For this review, take the finished solid that the model builds, in its own axes (mm). Face numbers are marked on the shaded views. A direction names the side the tool comes from. Coordinates: 2 decimals unless noted, no trailing zeros. Write each loop counter-clockwise with the first axis right and the second up, starting at its lowest first coordinate (ties: lowest second). Pieces come first, ordered by that corner, then holes.
1) We need section B-B on x = 40. Write out the cut boundary in (y, z).
2) Insertion check: P1, Ø5, axis at x = 164.5, y = 26.5, coming from the -Z side; P2, Ø5, axis at x = 167, z = 41.5, coming from the +Y side; P3, Ø3, axis at x = 5.5, y = 27, coming from the +Z side. Each pin has a flat end and moves straight along its axis. Give the tip position at first contact, or say it passes through.
3) For the marked faces 1 and 2, list the 3-axis set-ups (+Z, -Z, +X, -X, +Y, -Y) from which the entire face can be reached by the end or side of a thin tool; tool diameter is ignored.
4) We need section D-D on x = 109. Write out the cut boundary in (y, z), then the cut area to 3 significant figures.
5) Mouldability with a two-part tool opening along X and no side actions: class the marked faces 3, 4 and 5 as pulls with the +X half, pulls with the -X half, needs draft (parallel to the pull), parting line crosses it, or undercut.
6) To check wall thickness, follow line 1 along X through (y, z) = (87.5, 41); line 2 along Y through (x, z) = (120, 45). State the ranges of each line that lie inside material, in increasing order.
7) We need section A-A on y = 109. Write out the cut boundary in (x, z), then the cut area to 3 significant figures.
8) We need section C-C on z = 53. Write out the cut boundary in (x, y).
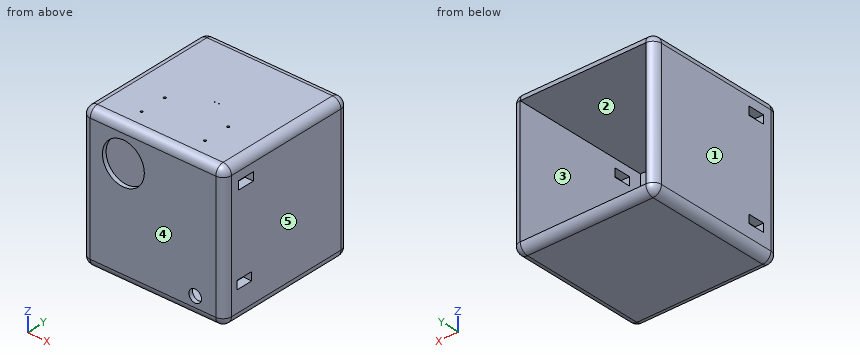
from build123d import *

# Parameters (mm, degrees)
SKETCH1_W           = 170
SKETCH1_H           = 170
BOSS_EXTRUDE2_DEPTH = 170
FILLET5_R           = 10
SKETCH6_W           = 150
SKETCH6_H           = 150
CUT_EXTRUDE2_DEPTH  = 165
SKETCH7_R           = 25
CUT_EXTRUDE3_DEPTH  = 5
SKETCH8_R           = 0.5
CUT_EXTRUDE4_DEPTH  = 5
SKETCH9_R           = 7.5
CUT_EXTRUDE5_DEPTH  = 5
SKETCH10_R          = 1.4
CUT_EXTRUDE8_DEPTH  = 5
SKETCH19_W          = 10
SKETCH19_H          = 20
CUT_EXTRUDE12_DEPTH = 15
SKETCH14_W          = 10
SKETCH14_H          = 20
CUT_EXTRUDE15_DEPTH = 15
SKETCH14_5_W        = 10
SKETCH14_5_H        = 20
CUT_EXTRUDE16_DEPTH = 15


with BuildPart() as part:
    # Sketch1 → Boss-Extrude2 (new body)
    with BuildSketch(Plane.XY):
        with Locations((85, 85)):
            Rectangle(SKETCH1_W, SKETCH1_H)
    extrude(amount=BOSS_EXTRUDE2_DEPTH)

    # Fillet5
    fillet5_edges = [part.edges().sort_by_distance(p)[0] for p in [
        (170, 85, 170),
        (85, 170, 170),
        (0, 85, 170),
        (85, 170, 0),
        (170, 85, 0),
        (85, 0, 0),
        (0, 85, 0),
        (0, 170, 85),
        (170, 170, 85),
        (170, 0, 85),
        (0, 0, 85),
        (85, 0, 170),
    ]]
    fillet(fillet5_edges, radius=FILLET5_R)

    # Sketch6 → Cut-Extrude2 (cut)
    with BuildSketch(Plane(origin=(0, 170, 0), x_dir=(1, 0, 0), z_dir=(0, 1, 0))):
        with Locations((85, -85)):
            Rectangle(SKETCH6_W, SKETCH6_H)
    extrude(amount=-CUT_EXTRUDE2_DEPTH, mode=Mode.SUBTRACT)

    # Sketch7 → Cut-Extrude3 (cut)
    with BuildSketch(Plane(origin=(0, 0, 0), x_dir=(-1, 0, 0), z_dir=(0, -1, 0))):
        with Locations(Location((-49.635709215, -128.113207768, 0), (0, 0, 90))):
            Circle(SKETCH7_R)
    extrude(amount=-CUT_EXTRUDE3_DEPTH, mode=Mode.SUBTRACT)

    # Sketch8 → Cut-Extrude4 (cut)
    with BuildSketch(Plane.XY.offset(170)):
        with Locations((87.027102924, 82.292149715)):
            Circle(SKETCH8_R)
        with Locations((92.027102924, 82.259165374)):
            Circle(SKETCH8_R)
    extrude(amount=-CUT_EXTRUDE4_DEPTH, mode=Mode.SUBTRACT)

    # Sketch9 → Cut-Extrude5 (cut)
    with BuildSketch(Plane(origin=(0, 0, 0), x_dir=(-1, 0, 0), z_dir=(0, -1, 0))):
        with Locations(Location((-135.371528781, -22.567188871, 0), (0, 0, 90))):
            Circle(SKETCH9_R)
    extrude(amount=-CUT_EXTRUDE5_DEPTH, mode=Mode.SUBTRACT)

    # Sketch10 → Cut-Extrude8 (cut)
    with BuildSketch(Plane.XY.offset(170)):
        with Locations((48.382145487, 58.196404185)):
            Circle(SKETCH10_R)
        with Locations((123.782145487, 58.455011456)):
            Circle(SKETCH10_R)
        with Locations((48.166639428, 26.796404185)):
            Circle(SKETCH10_R)
        with Locations((123.566639428, 27.055011456)):
            Circle(SKETCH10_R)
    extrude(amount=-CUT_EXTRUDE8_DEPTH, mode=Mode.SUBTRACT)

    # Sketch19 → Cut-Extrude12 (cut)
    with BuildSketch(Plane(origin=(170, 0, 0), x_dir=(0, 0, -1), z_dir=(1, 0, 0))):
        with Locations((-40, 27.793299749)):
            Rectangle(SKETCH19_W, SKETCH19_H)
        with Locations((-145, 30)):
            Rectangle(SKETCH19_W, SKETCH19_H)
    extrude(amount=-CUT_EXTRUDE12_DEPTH, mode=Mode.SUBTRACT)

    # Sketch14 → Cut-Extrude15 (cut)
    with BuildSketch(Plane.ZY):
        with Locations((30, 30)):
            Rectangle(SKETCH14_W, SKETCH14_H)
    extrude(amount=-CUT_EXTRUDE15_DEPTH, mode=Mode.SUBTRACT)

    # Sketch14_5 → Cut-Extrude16 (cut)
    with BuildSketch(Plane.ZY):
        with Locations((30, 30)):
            Rectangle(SKETCH14_5_W, SKETCH14_5_H)
        with Locations((145, 30)):
            Rectangle(SKETCH14_5_W, SKETCH14_5_H)
    extrude(amount=-CUT_EXTRUDE16_DEPTH, mode=Mode.SUBTRACT)


solid = part.part
Result:
1. outline: (0, 10) arc R10 ccw to (10, 0) - (160, 0) arc R10 ccw to (170, 10) - (5, 10) - (5, 105.04) - (0, 105.04) - close; (0, 151.18) - (5, 151.18) - (5, 160) - (170, 160) arc R10 ccw to (160, 170) - (10, 170) arc R10 ccw to (0, 160) - close
2. P1: stops at z = 0.2
2. P2: stops at y = 168.93
2. P3: stops at z = 169.54
3. face 1: +Z, -Z, -X, +Y, -Y
3. face 2: +Y
4. outline: (0, 10) arc R10 ccw to (10, 0) - (160, 0) arc R10 ccw to (170, 10) - (5, 10) - (5, 160) - (170, 160) arc R10 ccw to (160, 170) - (10, 170) arc R10 ccw to (0, 160) - close
4. area: 4,060 mm2
5. face 3: undercut
5. face 4: needs draft
5. face 5: pulls with the +X half
6. line 1: x = 0 to 10, 160 to 170
6. line 2: y = 0 to 5
7. outline: (0, 10) arc R10 ccw to (10, 0) - (160, 0) arc R10 ccw to (170, 10) - (170, 160) arc R10 ccw to (160, 170) - (10, 170) arc R10 ccw to (0, 160) - close; hole (10, 10) - (160, 10) - (160, 160) - (10, 160) - close
7. area: 6,310 mm2
8. outline: (0, 10) arc R10 ccw to (10, 0) - (160, 0) arc R10 ccw to (170, 10) - (170, 160) arc R10 ccw to (160, 170) - (160, 5) - (10, 5) - (10, 170) arc R10 ccw to (0, 160) - close
